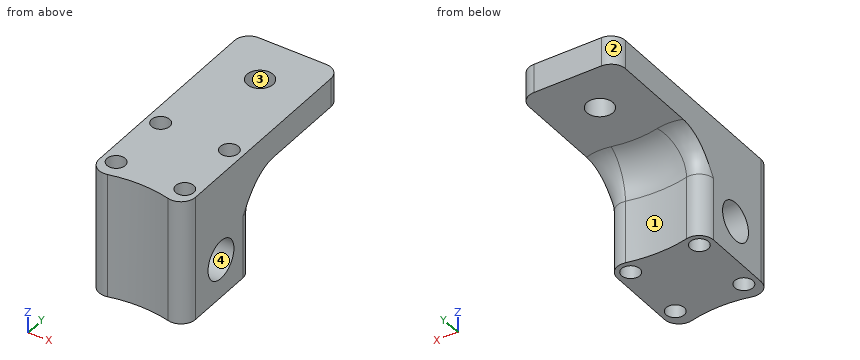
from build123d import *

# Parameters (mm, degrees)
F0_W         = 20
F0_H         = 22.7722101178
F0_R         = 1.8861050589
F0_H_2       = 26.2277898822
F0_R_2       = 2.7
F1_DEPTH     = 6
F2_DEPTH     = 20
F3_R         = 4
F4_DEPTH     = 25
F6_DEPTH     = 20
F7_DEPTH     = 26.001
F8_R         = 3
F9_T2_ANGLE  = 25.7767353783
F9_T6_ANGLE  = 359.64
F9_T11_ANGLE = 359.64


# Not quite as in the source:
# - a fillet or chamfer that OpenCascade refuses, or shapes differently, is made with other operations: its cross-section is extruded or revolved along the edge and cut away or added


with BuildPart() as f1:
    # F0 (on Top) → F1 (new body)
    with BuildSketch(Plane.XY):
        with Locations((0, -13.1138949411)):
            Rectangle(F0_W, F0_H)
        with Locations((-7.1138949411, -19.3861050589)):
            Circle(F0_R, mode=Mode.SUBTRACT)
        with Locations((-7.1138949411, -5.6138949411)):
            Circle(F0_R, mode=Mode.SUBTRACT)
        with Locations((7.1138949411, -19.3861050589)):
            Circle(F0_R, mode=Mode.SUBTRACT)
        with Locations((7.1138949411, -5.6138949411)):
            Circle(F0_R, mode=Mode.SUBTRACT)
        with Locations((0, 11.3861050589)):
            Rectangle(F0_W, F0_H_2)
        with Locations((0, 14.5)):
            Circle(F0_R_2, mode=Mode.SUBTRACT)
    extrude(amount=F1_DEPTH)

    # F0 (on Top) → F2 (join)
    with BuildSketch(Plane.XY):
        with Locations((0, -13.1138949411)):
            Rectangle(F0_W, F0_H)
        with Locations((-7.1138949411, -19.3861050589)):
            Circle(F0_R, mode=Mode.SUBTRACT)
        with Locations((-7.1138949411, -5.6138949411)):
            Circle(F0_R, mode=Mode.SUBTRACT)
        with Locations((7.1138949411, -19.3861050589)):
            Circle(F0_R, mode=Mode.SUBTRACT)
        with Locations((7.1138949411, -5.6138949411)):
            Circle(F0_R, mode=Mode.SUBTRACT)
    extrude(amount=-F2_DEPTH)

    # F3 (on face) → F4 (cut)
    with BuildSketch(Plane.YZ.offset(10)):
        with Locations((-12.5, -12)):
            Circle(F3_R)
    extrude(amount=-F4_DEPTH, mode=Mode.SUBTRACT)

    # F5 (on face) → F6 (cut, through all)
    with BuildSketch(Plane(origin=(0, 0, -20), x_dir=(1, 0, 0), z_dir=(0, 0, -1))):
        with BuildLine():
            Line((-10, 1.7277898822), (10, 1.7277898822))
            ThreePointArc((10, 1.7277898822), (0, 3.5477721311), (-10, 1.7277898822))
        make_face()
    extrude(amount=-F6_DEPTH, mode=Mode.SUBTRACT)

    # F5 (on face) → F7 (cut, through all)
    with BuildSketch(Plane(origin=(0, 0, -20), x_dir=(1, 0, 0), z_dir=(0, 0, -1))):
        with BuildLine():
            ThreePointArc((-10, 24.5), (0, 22.5), (10, 24.5))
            Line((10, 24.5), (-10, 24.5))
        make_face()
    extrude(amount=-F7_DEPTH, mode=Mode.SUBTRACT)

    # F8
    f8_edges = [f1.edges().sort_by_distance(p)[0] for p in [
        (-10, 24.5, 3),
        (10, 24.5, 3),
        (10, -24.5, -7),
        (-10, -24.5, -7),
        (-10, -1.72779, -10),
        (10, -1.72779, -10),
    ]]
    fillet(f8_edges, radius=F8_R)

    # F9: fillet of radius 7 on 1 edges, made by hand

    # F9_s1 → F9_t2 (revolve)
    with BuildSketch(Plane(origin=(5.3999454097, 1.2355988362, 0), x_dir=(0, 0, 1), z_dir=(0.9748064988, 0.2230522133, 0))):
        with BuildLine():
            ThreePointArc((0.0004, -2.8275125891), (-2.0502525317, 2.1232005646), (-7.0009656854, 4.1738530963))
            Line((-7.0009656854, 4.1738530963), (-7.0009656854, 4.8739896648))
            ThreePointArc((-7.0009656854, 4.8739896648), (-3.5004828427, 4.8735896648), (0, 4.8735896648))
            Line((0, 4.8735896648), (0.7001365685, 4.1734530963))
            ThreePointArc((0.7001365685, 4.1734530963), (0.7001365685, 0.6729702536), (0.7005365685, -2.8275125891))
            Line((0.7005365685, -2.8275125891), (0.0004, -2.8275125891))
        make_face()
    revolve(axis=Axis((0, 24.8350144179, 0), (0, 0, -1)), revolution_arc=F9_T2_ANGLE)


with BuildPart() as f9_tool4:
    # F9_s5 → F9_t6 (revolve)
    with BuildSketch(Plane(origin=(5.3999454097, 1.2355988362, 0), x_dir=(0, 0, 1), z_dir=(-0.9748064988, -0.2230522133, 0))):
        with BuildLine():
            ThreePointArc((0.0004, 2.8275125891), (-2.0502525317, -2.1232005646), (-7.0009656854, -4.1738530963))
            Line((-7.0009656854, -4.1738530963), (-7.0009656854, -4.8739896648))
            ThreePointArc((-7.0009656854, -4.8739896648), (-3.5004828427, -4.8735896648), (0, -4.8735896648))
            Line((0, -4.8735896648), (0.7001365685, -4.1734530963))
            ThreePointArc((0.7001365685, -4.1734530963), (0.7001365685, -0.6729702536), (0.7005365685, 2.8275125891))
            Line((0.7005365685, 2.8275125891), (0.0004, 2.8275125891))
        make_face()
    revolve(axis=Axis((7, -5.757129861, 0), (0, 0, -1)), revolution_arc=F9_T6_ANGLE)

    split(bisect_by=Plane.YZ.offset(10), keep=Keep.BOTTOM)


with BuildPart() as f1_1:
    add(f1.part)

    # F9_t3: union F9_tool4
    add(f9_tool4.part)


with BuildPart() as f9_tool9:
    # F9_s10 → F9_t11 (revolve)
    with BuildSketch(Plane(origin=(-5.348096652, 1.2591487889, 0), x_dir=(0, 0, 1), z_dir=(-0.9733857878, 0.22917266, 0))):
        with BuildLine():
            ThreePointArc((0.0004, 2.79284868), (-2.0502525317, -2.1578644738), (-7.0009656854, -4.2085170055))
            Line((-7.0009656854, -4.2085170055), (-7.0009656854, -4.908653574))
            ThreePointArc((-7.0009656854, -4.908653574), (-3.5004828427, -4.908253574), (0, -4.908253574))
            Line((0, -4.908253574), (0.7001365685, -4.2081170055))
            ThreePointArc((0.7001365685, -4.2081170055), (0.7001365685, -0.7076341628), (0.7005365685, 2.79284868))
            Line((0.7005365685, 2.79284868), (0.0004, 2.79284868))
        make_face()
    revolve(axis=Axis((-7, -5.757129861, 0), (0, 0, -1)), revolution_arc=F9_T11_ANGLE)

    split(bisect_by=Plane.YZ.offset(-10), keep=Keep.TOP)


with BuildPart() as f1_2:
    add(f1_1.part)

    # F9_t8: union F9_tool9
    add(f9_tool9.part)


solid = f1_2.part
Design review of the part built by this model. Coordinates are the model's own, in mm. Face numbers are marked on the shaded views. Coordinates: 2 decimals unless noted, no trailing zeros. Write each loop counter-clockwise with the first axis right and the second up, starting at its lowest first coordinate (ties: lowest second). Pieces come first, ordered by that corner, then holes. Notation, with made-up numbers: (-29.5, 72.25) - (-25.5, 72.25) arc R19 ccw to (-25.5, 98.25) - close; hole circle Ø3 at (32, 7.5). An arc over 180 degrees is marked (long way). Use one line per item in the form item = value.
Q1. Consider section B-B (y = 14.5). Write out the cut boundary in (x, z).
Taken from the geometry:
outline = (-10, 0) - (-2.7, 0) - (-2.7, 6) - (-10, 6) - close; (2.7, 0) - (10, 0) - (10, 6) - (2.7, 6) - close
Q2. Consider section D-D (y = -18). Write out the cut boundary in (x, z).
Taken from the geometry:
outline = (-10, -20) - (-8.39, -20) - (-8.39, 6) - (-10, 6) - close; (-5.83, -20) - (5.83, -20) - (5.83, 6) - (-5.83, 6) - close; (8.39, -20) - (10, -20) - (10, 6) - (8.39, 6) - close
Q3. For probe 1 along X at (y, z) = (-19.5, 0); probe 2 along Y at (x, z) = (-7.25, 3); probe 3 along Y at (x, z) = (8.25, -12.5), list the stretches that pass through material, from the lowest coordinate up.
Taken from the geometry:
probe_1 = -10 to -9, -5.23 to 5.23, 9 to 10
probe_2 = -23.35 to -21.27, -17.5 to -7.5, -3.73 to 24.49
probe_3 = -23.08 to -20.89, -17.88 to -16.47, -8.53 to -7.12, -4.11 to -3.03
Q4. Consider section A-A (x = 0). Write out the cut boundary in (y, z), plus the area to 3 significant figures.
Taken from the geometry:
outline = (-22.5, -20) - (-3.55, -20) - (-3.55, -6.93) arc R7 cw to (3.38, 0) - (11.8, 0) - (11.8, 6) - (-22.5, 6) - close; (17.2, 0) - (24.5, 0) - (24.5, 6) - (17.2, 6) - close; hole circle Ø8 at (-12.5, -12)
area = 589 mm^2
Q5. The part is to be moulded in two halves that separate along X. For the marked faces 1, 2, 3 and 4, say which applies: +X half, -X half, draft (parallel to the pull), parting line (faces both ways), or undercut.
Taken from the geometry:
face_1 = undercut
face_2 = -X half
face_3 = undercut
face_4 = draft
Q6. Consider section C-C (z = -10.75). Write out the cut boundary in (x, y), plus the area to 3 significant figures.
Taken from the geometry:
outline = (-10, -20.36) arc R3 ccw to (-6.28, -23.27) arc R26 cw to (6.28, -23.27) arc R3 ccw to (10, -20.36) - (10, -16.3) - (-10, -16.3) - close; (-10, -8.7) - (10, -8.7) - (10, -5.76) arc R3 ccw to (6.33, -2.83) arc R28.38 cw to (-6.33, -2.83) arc R3 ccw to (-10, -5.76) - close; hole circle Ø3.77 at (-7.11, -19.39); hole circle Ø3.77 at (-7.11, -5.61); hole circle Ø3.77 at (7.11, -19.39); hole circle Ø3.77 at (7.11, -5.61)
area = 193 mm^2
Q7. Insertion check: pin 1 Ø2.5 at (x, y) = (-7.11, -19.39) entering from +Z; pin 2 Ø6 at (x, y) = (-1, 9) entering from -Z; pin 3 Ø10 at (x, z) = (-2.5, 1.5) entering from -Y; pin 4 Ø1.5 at (x, z) = (4, -16) entering from +Y. Each pin has a flat end and moves straight along its axis. Give the tip position at first contact, or say it passes through.
Taken from the geometry:
pin_1 = through
pin_2 = 0
pin_3 = -23.36
pin_4 = -3.15
